Could you check a few things on this model? Use its own coordinates, in mm. Round coordinates to 2 decimals unless told otherwise and drop trailing zeros. Order: outer loops, then holes, each group sorted by start corner. A loop starts at its lowest first (then second) coordinate and runs counter-clockwise, first axis right, second up. Notation, with made-up numbers: (-14, 7.25) - (12, 7.25) arc R27 ccw to (12, 45.25) - close; hole circle Ø9 at (-27, 60.5). An arc over 180 degrees is marked (long way). Use one line per item in the form item = value.
Solid Edge part; units mm, degrees
sketch "Sketch1" plane through (0, 0, 0) normal (0, 0, 1) x (1, 0, 0)
  line L0 (-250, -144.3376) -> (250, -144.3376)
  line L1 (250, -144.3376) -> (0, 288.6751)
  line L2 (0, 288.6751) -> (-250, -144.3376)
extrude "Protrusion1" add sketch "Sketch1" along normal up to vertex (408.2483 mm away)
sketch "Sketch2" plane through (0, 0, 0) normal (1, 0, 0) x (0, 1, 0)
  line L0 (0, 408.2483) -> (-144.3376, 0)
extrude "Cutout1" cut sketch "Sketch2" against normal up to next and the other way up to next material side at (0, -72.2159, 204.1408)
pattern_circular "Pattern1" count 3 over 360 about axis through (0, 0, 408.2483) along (0, 0, -1) of "Cutout1"
Item 1: Imagine slicing it at B-B on z = 316.5. Please give me the cut outline in (x, y).
Found:
outline = (-56.18, -32.44) - (56.18, -32.44) - (0, 64.88) - close
Item 2: Will these pins go through, and if not, where does the flat tip stop? P1, Ø4, axis at y = 19.5, z = 332, coming from the +X side; P2, Ø8, axis at x = 49.5, z = 325.5, coming from the +Y side; P3, Ø8, axis at x = 20.5, z = 237, coming from the +Y side.
Found:
P1 = 21.28
P2 = -19.74
P3 = 93.07
Item 3: I need wall thicknesses on L1, parallel to X at y = 125, z = 129.5; L2, parallel to Y at x = 83, z = 183.5; L3, parallel to Y at x = -17, z = 351. Which ranges of each line are inside material? Lowest first, please.
Found:
L1 = -41.63 to 41.63
L2 = -79.46 to 15.16
L3 = -20.24 to 11.04
